The listing builds one solid part. Answer for the finished solid, in the listing's coordinates (mm). A direction names the side the tool comes from. Coordinates: 2 decimals unless noted, no trailing zeros. Write each loop counter-clockwise with the first axis right and the second up, starting at its lowest first coordinate (ties: lowest second). Pieces come first, ordered by that corner, then holes.
```python
from build123d import *

# Parameters (mm, degrees)
F0_R     = 2.6
F0_R_2   = 1.55
F1_DEPTH = 12
F2_R     = 4.225
F3_DEPTH = 7
F5_DEPTH = 4


with BuildPart() as f1:
    # F0 (on Top) → F1 (new body)
    with BuildSketch(Plane.XY):
        with BuildLine():
            ThreePointArc((-30.82763, 20.107742), (-32.912276, 22.00702), (-34.013815, 24.603098))
            ThreePointArc((-34.013815, 24.603098), (-43.8, 29.098454), (-44.8, 18.375691))
            ThreePointArc((-44.8, 18.375691), (-43.102501, 16.123691), (-42.5, 13.368696))
            Line((-42.5, 13.368696), (-42.5, -13.368696))
            ThreePointArc((-42.5, -13.368696), (-43.102501, -16.123691), (-44.8, -18.375691))
            ThreePointArc((-44.8, -18.375691), (-43.8, -29.098454), (-34.013815, -24.603098))
            ThreePointArc((-34.013815, -24.603098), (-32.912276, -22.00702), (-30.82763, -20.107742))
            Line((-30.82763, -20.107742), (-18.561811, -13.026067))
            ThreePointArc((-18.561811, -13.026067), (-16.037247, -12.509627), (-13.707877, -13.611522))
            ThreePointArc((-13.707877, -13.611522), (-7.600624, -14.240378), (-5.487994, -8.475762))
            ThreePointArc((-5.487994, -8.475762), (-4.905969, -6.345122), (-2.722478, -6.01233))
            ThreePointArc((-2.722478, -6.01233), (6.6, 0), (-2.722478, 6.01233))
            ThreePointArc((-2.722478, 6.01233), (-4.905969, 6.345122), (-5.487994, 8.475762))
            ThreePointArc((-5.487994, 8.475762), (-7.600624, 14.240378), (-13.707877, 13.611522))
            ThreePointArc((-13.707877, 13.611522), (-16.619309, 13.081574), (-18.25, 15.551013))
            Line((-18.25, 15.551013), (-18.25, 23.382686))
            ThreePointArc((-18.25, 23.382686), (-17.664214, 24.796899), (-16.25, 25.382686))
            ThreePointArc((-16.25, 25.382686), (-13.95, 27.682686), (-16.25, 29.982686))
            Line((-16.25, 29.982686), (-24.25, 29.982686))
            ThreePointArc((-24.25, 29.982686), (-26.55, 27.682686), (-24.25, 25.382686))
            ThreePointArc((-24.25, 25.382686), (-22.835786, 24.796899), (-22.25, 23.382686))
            Line((-22.25, 23.382686), (-22.25, 19.80625))
            ThreePointArc((-22.25, 19.80625), (-23.592572, 17.480847), (-26.277716, 17.480847))
            Line((-26.277716, 17.480847), (-30.82763, 20.107742))
        make_face()
        with Locations((-40.5, -23.382686)):
            Circle(F0_R, mode=Mode.SUBTRACT)
        with Locations((-30.25, -10)):
            Circle(F0_R_2, mode=Mode.SUBTRACT)
        with BuildLine():
            ThreePointArc((-25.409667, 6.454415), (-22.637088, 8.243459), (-19.37854, 7.724104))
            Line((-19.37854, 7.724104), (-6.375, 0.216506))
            ThreePointArc((-6.375, 0.216506), (-6.25, 0), (-6.375, -0.216506))
            Line((-6.375, -0.216506), (-19.37854, -7.724104))
            ThreePointArc((-19.37854, -7.724104), (-22.637088, -8.243459), (-25.409667, -6.454415))
            ThreePointArc((-25.409667, -6.454415), (-30.25, -4), (-35.090333, -6.454415))
            ThreePointArc((-35.090333, -6.454415), (-36.580889, -6.933918), (-37.5, -5.666277))
            Line((-37.5, -5.666277), (-37.5, 5.666277))
            ThreePointArc((-37.5, 5.666277), (-36.580889, 6.933918), (-35.090333, 6.454415))
            ThreePointArc((-35.090333, 6.454415), (-30.25, 4), (-25.409667, 6.454415))
        make_face(mode=Mode.SUBTRACT)
        with Locations((-10.25, -10)):
            Circle(F0_R_2, mode=Mode.SUBTRACT)
        Circle(F0_R, mode=Mode.SUBTRACT)
        with Locations((-30.25, 10)):
            Circle(F0_R_2, mode=Mode.SUBTRACT)
        with Locations((-40.5, 23.382686)):
            Circle(F0_R, mode=Mode.SUBTRACT)
        with Locations((-10.25, 10)):
            Circle(F0_R_2, mode=Mode.SUBTRACT)
    extrude(amount=F1_DEPTH)

    # F2 (on face) → F3 (cut)
    with BuildSketch(Plane.XY.offset(12)):
        with Locations((-40.5, 23.382686)):
            Circle(F2_R)
        Circle(F2_R)
        with Locations((-40.5, -23.382686)):
            Circle(F2_R)
    extrude(amount=-F3_DEPTH, mode=Mode.SUBTRACT)

    # F4 (on face) → F5 (cut)
    with BuildSketch(Plane(origin=(0, 0, 0), x_dir=(1, 0, 0), z_dir=(0, 0, -1))):
        Polygon((-27.45, 8.383419), (-27.45, 11.616581), (-30.25, 13.233162), (-33.05, 11.616581), (-33.05, 8.383419), (-30.25, 6.766838), align=None)
        Polygon((-27.45, -11.616581), (-27.45, -8.383419), (-30.25, -6.766838), (-33.05, -8.383419), (-33.05, -11.616581), (-30.25, -13.233162), align=None)
        Polygon((-13.05, -8.383419), (-13.05, -11.616581), (-10.25, -13.233162), (-7.45, -11.616581), (-7.45, -8.383419), (-10.25, -6.766838), align=None)
        Polygon((-13.05, 11.616581), (-13.05, 8.383419), (-10.25, 6.766838), (-7.45, 8.383419), (-7.45, 11.616581), (-10.25, 13.233162), align=None)
    extrude(amount=-F5_DEPTH, mode=Mode.SUBTRACT)


solid = f1.part
```
(1) Section B-B, the plane x = 0 is taken. Write down the section's boundary in (y, z) (3 decimals).
(2) Section A-A, the plane y = -10 is taken. Write down the section's boundary in (x, z).
(3) Section C-C, the plane x = -40.5 is taken. Write down the section's boundary in (y, z), plus the area to 3 significant figures.
(4) Find the intervals of material crossed by probe 1 along X at (y, z) = (10, 6); probe 2 along Y at (x, z) = (-40.5, 3.1); probe 3 along Y at (x, z) = (-30.5, 9.75), in increasing order.
(5) Section D-D, the plane z = 8.5 is taken. State how many separate pieces and enclosed holes the cut face has, plus the area to 3 significant figures.
(6) For a pull along Y with two mould halves and no side action, classify faces 1 (the flat face through (-24.781, -16.616, 5.916)), 2 (the flat face through (-11.63, -12.436, 1.972)) as pulls with the +Y half, pulls with the -Y half, needs draft (parallel to the pull), parting line crosses it, or undercut.
(7) Each of these flat-tipped pins is pushed along its axis until it touches: pin 1 (1 mm diameter, centred on x = -2.5, z = 10.5, fed in from -Y); pin 2 (1.6 mm diameter, centred on y = -10.5, z = 3, fed in from +X); pin 3 (1.9 mm diameter, centred on x = -30.25, y = 10, fed in from +Z); pin 4 (13.5 mm diameter, centred on x = -40.5, y = 23.38, fed in from -Z). Where does it stop, or does it pass through?
(8) Which of the six approach directions +Z, -Z, +X, -X, +Y, -Y give full straight-line access (tool end or side, diameter ignored) to faces 3 (the flat face through (-31.67, 12.414, 1.972)), 4 (the flat face through (-40.6, 20.6, 5)), 5 (the cylindrical face through (-36.603, 6.926, 5.916)), 6 (the flat face through (-42.5, 0, 6))?
Solution:
1. outline: (-6.6, 0) - (-2.6, 0) - (-2.6, 5) - (-4.225, 5) - (-4.225, 12) - (-6.6, 12) - close; (2.6, 0) - (6.6, 0) - (6.6, 12) - (4.225, 12) - (4.225, 5) - (2.6, 5) - close
2. outline: (-42.5, 0) - (-33.05, 0) - (-33.05, 4) - (-31.8, 4) - (-31.8, 12) - (-42.5, 12) - close; (-28.7, 4) - (-27.45, 4) - (-27.45, 0) - (-13.05, 0) - (-13.05, 4) - (-11.8, 4) - (-11.8, 12) - (-28.7, 12) - close; (-8.7, 4) - (-7.45, 4) - (-7.45, 0) - (-5.25, 0) - (-5.25, 12) - (-8.7, 12) - close
3. outline: (-29.98, 0) - (-25.98, 0) - (-25.98, 5) - (-27.61, 5) - (-27.61, 12) - (-29.98, 12) - close; (-20.78, 0) - (20.78, 0) - (20.78, 5) - (19.16, 5) - (19.16, 12) - (-19.16, 12) - (-19.16, 5) - (-20.78, 5) - close; (25.98, 0) - (29.98, 0) - (29.98, 12) - (27.61, 12) - (27.61, 5) - (25.98, 5) - close
3. area: 549 mm2
4. probe 1: x = -42.5 to -31.8, -28.7 to -11.8, -8.7 to -5.25
4. probe 2: y = -29.98 to -25.98, -20.78 to 20.78, 25.98 to 29.98
4. probe 3: y = -19.92 to -11.53, -8.47 to -4.01, 4.01 to 8.47, 11.53 to 19.92
5. separate pieces: 1
5. enclosed holes: 8
5. area: 1,210 mm2
6. face 1: pulls with the -Y half
6. face 2: undercut
7. pin 1: stops at y = -6.29
7. pin 2: stops at x = -5.25
7. pin 3: passes through
7. pin 4: stops at z = 0
8. face 3: -Z
8. face 4: +Z
8. face 5: +Z, -Z
8. face 6: +Z, -Z, -X
